Here's how the part is built. I have some questions about the finished solid (model axes, mm). A direction names the side the tool comes from. Give positions to 0.01 mm unless a question says otherwise; leave off trailing zeros. Loops run counter-clockwise (first coordinate to the right, second up) from the corner with the lowest first, then second, coordinate; pieces in that order, holes last.
Q1. We'd pull the mould along Y, two halves only. Please class faces 4 (the face through (10.734, 7.768, 1.972)), 5 (the face through (4.1, -12.6, 2)), 6 (the face through (-6.348, 12.478, 1.972)): +Y half, -Y half, draft (parallel to the pull), parting line (faces both ways), or undercut.
Q2. If we section it at A-A (y = 8): Please give me the cut outline in (x, z).
Q3. Will these pins go through, and if not, where does the flat tip stop? P1, Ø2, axis at x = 10.5, z = 2.5, coming from the -Y side; P2, Ø2, axis at y = 7, z = 2, coming from the -X side; P3, Ø1.5, axis at x = -7.5, z = 1, coming from the -Y side.
Q4. I need wall thicknesses on line 1 (Z direction, x = -2.5, y = -11.75); line 2 (Y direction, x = 2.75, z = 0.85); line 3 (X direction, y = 3.5, z = 4.25). Which ranges of each line are inside material? Lowest first, please.
Q5. If we section it at B-B (x = 11.75): Please give me the cut outline in (y, z), plus the area to 3 significant figures.
Q6. For faces 1 (the face through (-12.478, -6.348, 1.972)), 2 (the face through (2, 3.52, 2.22)), 3 (the face through (6, -3, 4)), which set-ups out of +Z, -Z, +X, -X, +Y, -Y let a thin tool reach every point of the face, with its end or its side?
from build123d import *

# Parameters (mm, degrees)
F0_R     = 6.5
F1_DEPTH = 4
F2_DEPTH = 4.5


with BuildPart() as f1:
    # F0 (on Top) → F1 (new body)
    with BuildSketch(Plane.XY):
        with BuildLine():
            ThreePointArc((13.909274, -1.591255), (13.25, 0), (13.909274, 1.591255))
            ThreePointArc((13.909274, 1.591255), (13.827637, 2.190083), (13.720231, 2.784829))
            ThreePointArc((13.720231, 2.784829), (12.601499, 4.094475), (12.736781, 5.811575))
            ThreePointArc((12.736781, 5.811575), (12.474091, 6.355867), (12.188155, 6.888314))
            ThreePointArc((12.188155, 6.888314), (10.719475, 7.788155), (10.317523, 9.463018))
            ThreePointArc((10.317523, 9.463018), (9.899495, 9.899495), (9.463018, 10.317523))
            ThreePointArc((9.463018, 10.317523), (7.788155, 10.719475), (6.888314, 12.188155))
            ThreePointArc((6.888314, 12.188155), (6.355867, 12.474091), (5.811575, 12.736781))
            ThreePointArc((5.811575, 12.736781), (4.094475, 12.601499), (2.784829, 13.720231))
            ThreePointArc((2.784829, 13.720231), (2.190083, 13.827637), (1.591255, 13.909274))
            ThreePointArc((1.591255, 13.909274), (0, 13.25), (-1.591255, 13.909274))
            ThreePointArc((-1.591255, 13.909274), (-2.190083, 13.827637), (-2.784829, 13.720231))
            ThreePointArc((-2.784829, 13.720231), (-4.094475, 12.601499), (-5.811575, 12.736781))
            ThreePointArc((-5.811575, 12.736781), (-6.355867, 12.474091), (-6.888314, 12.188155))
            ThreePointArc((-6.888314, 12.188155), (-7.788155, 10.719475), (-9.463018, 10.317523))
            ThreePointArc((-9.463018, 10.317523), (-9.899495, 9.899495), (-10.317523, 9.463018))
            ThreePointArc((-10.317523, 9.463018), (-10.296714, 9.287391), (-10.289763, 9.110671))
            ThreePointArc((-10.289763, 9.110671), (-10.828971, 7.649271), (-12.188155, 6.888314))
            ThreePointArc((-12.188155, 6.888314), (-12.474091, 6.355867), (-12.736781, 5.811575))
            ThreePointArc((-12.736781, 5.811575), (-12.553587, 5.315197), (-12.491376, 4.789763))
            ThreePointArc((-12.491376, 4.789763), (-12.823033, 3.613982), (-13.720231, 2.784829))
            ThreePointArc((-13.720231, 2.784829), (-13.827637, 2.190083), (-13.909274, 1.591255))
            ThreePointArc((-13.909274, 1.591255), (-13.421343, 0.86121), (-13.25, 0))
            ThreePointArc((-13.25, 0), (-13.421343, -0.86121), (-13.909274, -1.591255))
            ThreePointArc((-13.909274, -1.591255), (-13.827637, -2.190083), (-13.720231, -2.784829))
            ThreePointArc((-13.720231, -2.784829), (-12.823033, -3.613982), (-12.491376, -4.789763))
            ThreePointArc((-12.491376, -4.789763), (-12.553587, -5.315197), (-12.736781, -5.811575))
            ThreePointArc((-12.736781, -5.811575), (-12.474091, -6.355867), (-12.188155, -6.888314))
            ThreePointArc((-12.188155, -6.888314), (-10.828971, -7.649271), (-10.289763, -9.110671))
            ThreePointArc((-10.289763, -9.110671), (-10.296714, -9.287391), (-10.317523, -9.463018))
            ThreePointArc((-10.317523, -9.463018), (-9.899495, -9.899495), (-9.463018, -10.317523))
            ThreePointArc((-9.463018, -10.317523), (-7.788155, -10.719475), (-6.888314, -12.188155))
            ThreePointArc((-6.888314, -12.188155), (-6.355867, -12.474091), (-5.811575, -12.736781))
            ThreePointArc((-5.811575, -12.736781), (-4.094475, -12.601499), (-2.784829, -13.720231))
            ThreePointArc((-2.784829, -13.720231), (-2.190083, -13.827637), (-1.591255, -13.909274))
            ThreePointArc((-1.591255, -13.909274), (0, -13.25), (1.591255, -13.909274))
            ThreePointArc((1.591255, -13.909274), (2.190083, -13.827637), (2.784829, -13.720231))
            ThreePointArc((2.784829, -13.720231), (4.094475, -12.601499), (5.811575, -12.736781))
            ThreePointArc((5.811575, -12.736781), (6.355867, -12.474091), (6.888314, -12.188155))
            ThreePointArc((6.888314, -12.188155), (7.788155, -10.719475), (9.463018, -10.317523))
            ThreePointArc((9.463018, -10.317523), (9.899495, -9.899495), (10.317523, -9.463018))
            ThreePointArc((10.317523, -9.463018), (10.719475, -7.788155), (12.188155, -6.888314))
            ThreePointArc((12.188155, -6.888314), (12.474091, -6.355867), (12.736781, -5.811575))
            ThreePointArc((12.736781, -5.811575), (12.601499, -4.094475), (13.720231, -2.784829))
            ThreePointArc((13.720231, -2.784829), (13.827637, -2.190083), (13.909274, -1.591255))
        make_face()
        Circle(F0_R, mode=Mode.SUBTRACT)
    extrude(amount=F1_DEPTH)

    # F0 (on Top) → F2 (join)
    with BuildSketch(Plane.XY):
        Circle(F0_R)
        Polygon((4.05, 2.338269), (4.05, -2.338269), (0, -4.676537), (-4.05, -2.338269), (-4.05, 2.338269), (0, 4.676537), align=None, mode=Mode.SUBTRACT)
    extrude(amount=F2_DEPTH)


solid = f1.part
Check sheet entries:
1. face 4: undercut
1. face 5: -Y half
1. face 6: +Y half
2. outline: (-10.58, 0) - (10.58, 0) - (10.58, 4) - (-10.58, 4) - close
3. P1: stops at y = -10.28
3. P2: stops at x = -12.65
3. P3: stops at y = -12.27
4. line 1: z = 0 to 4
4. line 2: y = -13.73 to -3.09, 3.09 to 13.73
4. line 3: x = -5.48 to -2.04, 2.04 to 5.48
5. outline: (-7, 0) - (7, 0) - (7, 4) - (-7, 4) - close
5. area: 56.0 mm2
6. face 1: +Z, -Z, -X, -Y
6. face 2: +Z, -Z
6. face 3: +Z
